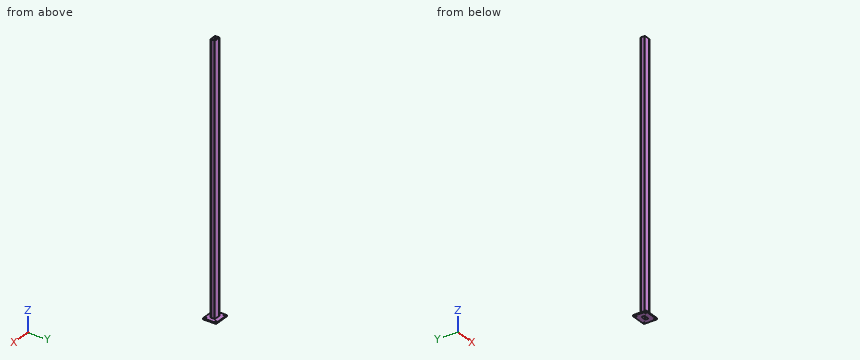
from build123d import *

# Parameters (mm, degrees)
F0_W     = 140
F0_H     = 120
F0_R     = 5.5
F1_DEPTH = 10
F2_DEPTH = 2400


with BuildPart() as f1:
    # F0 (on Top) → F1 (new body)
    with BuildSketch(Plane.XY):
        Rectangle(F0_W, F0_H)
        with Locations((-55, -45)):
            Circle(F0_R, mode=Mode.SUBTRACT)
        with Locations((55, -45)):
            Circle(F0_R, mode=Mode.SUBTRACT)
        with Locations((-55, 45)):
            Circle(F0_R, mode=Mode.SUBTRACT)
        with BuildLine():
            ThreePointArc((-30, 15), (-28.535534, 18.535534), (-25, 20))
            Line((-25, 20), (25, 20))
            ThreePointArc((25, 20), (28.535534, 18.535534), (30, 15))
            Line((30, 15), (30, -15))
            ThreePointArc((30, -15), (28.535534, -18.535534), (25, -20))
            Line((25, -20), (-25, -20))
            ThreePointArc((-25, -20), (-28.535534, -18.535534), (-30, -15))
            Line((-30, -15), (-30, 15))
        make_face(mode=Mode.SUBTRACT)
        with Locations((55, 45)):
            Circle(F0_R, mode=Mode.SUBTRACT)
    extrude(amount=F1_DEPTH)

    # F0 (on Top) → F2 (join)
    with BuildSketch(Plane.XY):
        with BuildLine():
            Line((25, 20), (-25, 20))
            ThreePointArc((-25, 20), (-28.535534, 18.535534), (-30, 15))
            Line((-30, 15), (-30, -15))
            ThreePointArc((-30, -15), (-28.535534, -18.535534), (-25, -20))
            Line((-25, -20), (25, -20))
            ThreePointArc((25, -20), (28.535534, -18.535534), (30, -15))
            Line((30, -15), (30, 15))
            ThreePointArc((30, 15), (28.535534, 18.535534), (25, 20))
        make_face()
        with BuildLine():
            ThreePointArc((-25, 10), (-23.535534, 13.535534), (-20, 15))
            Line((-20, 15), (20, 15))
            ThreePointArc((20, 15), (23.535534, 13.535534), (25, 10))
            Line((25, 10), (25, -10))
            ThreePointArc((25, -10), (23.535534, -13.535534), (20, -15))
            Line((20, -15), (-20, -15))
            ThreePointArc((-20, -15), (-23.535534, -13.535534), (-25, -10))
            Line((-25, -10), (-25, 10))
        make_face(mode=Mode.SUBTRACT)
    extrude(amount=F2_DEPTH)


solid = f1.part
Read the model definition and answer for the solid it produces. Units are mm, in the model's axes. Round coordinates to 2 decimals unless told otherwise and drop trailing zeros. Write each loop counter-clockwise with the first axis right and the second up, starting at its lowest first coordinate (ties: lowest second). Pieces come first, ordered by that corner, then holes. Notation, with made-up numbers: M 71,-39.5 L 87,-39.5 A7 ccw 87,-29.5 Z; hole C -21,36 d5. An arc over 180 degrees is marked long. Use a Markdown table: item, result.
1) Flat-ended cylindrical pins translate along their axes: pin 1 (25 mm diameter, centred on x = -4, z = 1074.5, fed in from +Y); pin 2 (9 mm diameter, centred on y = 3, z = 1149, fed in from -X); pin 3 (24 mm diameter, centred on y = -7, z = 1793.5, fed in from +X); pin 4 (9 mm diameter, centred on x = -55, y = -45, fed in from +Z). Find the tip coordinate at first contact, or state that the pin passes through.
Answers follow:
| item | result |
|---|---|
| pin 1 | stops at y = 20 |
| pin 2 | stops at x = -30 |
| pin 3 | stops at x = 30 |
| pin 4 | passes through |
2) Straight lines are drawn through the part: line 1 along Y through (x, z) = (-55, 4.25); line 2 along Y through (x, z) = (10, 434.5); line 3 along X through (y, z) = (-2.5, 532.5). For each, find the intervals that lie inside material, in ascending order. Write a range as [from, to].
Answers follow:
| item | result |
|---|---|
| line 1 | y = [-60, -50.5], [-39.5, 39.5], [50.5, 60] |
| line 2 | y = [-20, -15], [15, 20] |
| line 3 | x = [-30, -25], [25, 30] |
3) The part is cut by section A-A (z = 1215.5). Write down the section's boundary in (x, y).
Answers follow:
| item | result |
|---|---|
| outline | M -30,-15 A5 ccw -25,-20 L 25,-20 A5 ccw 30,-15 L 30,15 A5 ccw 25,20 L -25,20 A5 ccw -30,15 Z; hole M -25,-10 A5 ccw -20,-15 L 20,-15 A5 ccw 25,-10 L 25,10 A5 ccw 20,15 L -20,15 A5 ccw -25,10 Z |
